Design review of the part built by this model. Coordinates are the model's own, in mm. Coordinates: 2 decimals unless noted, no trailing zeros. Order: outer loops, then holes, each group sorted by start corner. A loop starts at its lowest first (then second) coordinate and runs counter-clockwise, first axis right, second up. Notation, with made-up numbers: (72.5, 21) - (98.5, 21) arc R14 ccw to (98.5, 25) - close; hole circle Ø2 at (58.5, 1). An arc over 180 degrees is marked (long way). Write item = value, one per line. Start each with the question number.
```python
from build123d import *

# Parameters (mm, degrees)
F0_W     = 50.8
F0_H     = 50.8
F1_DEPTH = 6.35
F2_R     = 2.54
F4_D     = 7.9375


with BuildPart() as f1:
    # F0 (on Front) → F1 (new body)
    with BuildSketch(Plane.XZ):
        Rectangle(F0_W, F0_H)
    extrude(amount=F1_DEPTH)

    # F2
    f2_edges = [f1.edges().sort_by_distance(p)[0] for p in [
        (25.4, -6.35, 0),
        (0, -6.35, -25.4),
        (-25.4, -6.35, 0),
        (0, -6.35, 25.4),
    ]]
    fillet(f2_edges, radius=F2_R)

    # F4 (through all)
    with Locations(Plane.XZ.offset(6.35)):
        with Locations((0, 0)):
            Hole(F4_D / 2)


solid = f1.part
```
Item 1: Add section A-A on z = 0. Give the boundary of the cut face in (x, y).
Item 2: Add section C-C on y = -2.5. Give the boundary of the cut face in (x, z).
Item 3: For line 1 (Z direction, x = 0, y = -3.25); line 2 (X direction, y = -4, z = -7.5), list the stretches that pass through material, from the lowest coordinate up.
Item 4: Add section B-B on x = 0. Give the boundary of the cut face in (y, z).
Item 5: For P1, Ø1, axis at x = 12, y = -4.5, coming from the -Z side; P2, Ø1, axis at x = -2.5, y = -5, coming from the +Z side; P3, Ø7, axis at x = 0, z = 0, coming from the +Y side (3 decimals), all flat-tipped, find the tip position at first contact; note any pin that passes through.
Item 6: Mouldability with a two-part tool opening along X and no side actions: class faces 1 (the cylindrical face through (0.86, -3.131, -3.874)), 2 (the cylindrical face through (-24.676, -5.586, 0.356)), 3 (the cylindrical face through (0.356, -5.586, -24.676)) as +X half, -X half, draft (parallel to the pull), parting line (faces both ways), or undercut.
Worked out:
q1.outline = (-25.4, -3.81) arc R2.54 ccw to (-22.86, -6.35) - (-3.97, -6.35) - (-3.97, 0) - (-25.4, 0) - close; (3.97, -6.35) - (22.86, -6.35) arc R2.54 ccw to (25.4, -3.81) - (25.4, 0) - (3.97, 0) - close
q2.outline = (-25.4, -25.4) - (25.4, -25.4) - (25.4, 25.4) - (-25.4, 25.4) - close; hole circle Ø7.94 at (0, 0)
q3.line_1 = -25.4 to -3.97, 3.97 to 25.4
q3.line_2 = -25.39 to 25.39
q4.outline = (-6.35, -22.86) arc R2.54 ccw to (-3.81, -25.4) - (0, -25.4) - (0, -3.97) - (-6.35, -3.97) - close; (-6.35, 3.97) - (0, 3.97) - (0, 25.4) - (-3.81, 25.4) arc R2.54 ccw to (-6.35, 22.86) - close
q5.P1 = -25.39
q5.P2 = 25.3
q5.P3 = through
q6.face_1 = undercut
q6.face_2 = -X half
q6.face_3 = draft
